For this review, take the finished solid that the model builds, in its own axes (mm). A direction names the side the tool comes from. Coordinates: 2 decimals unless noted, no trailing zeros. Order: outer loops, then holes, each group sorted by start corner. A loop starts at its lowest first (then second) coordinate and runs counter-clockwise, first axis right, second up. Notation, with made-up numbers: M 58,-24.75 L 73,-24.75 A20 ccw 73,3.25 Z; hole C -16,82.25 d4. An arc over 180 degrees is marked long. Use CSV: the item, a comma, the result in double quotes.
Autodesk Inventor part; units mm, degrees
ref_plane "YZ Plane" through (0, 0, 0) normal (1, 0, 0) x (0, 1, 0)
ref_plane "XZ Plane" through (0, 0, 0) normal (0, 1, 0) x (-1, 0, 0)
ref_plane "XY Plane" through (0, 0, 0) normal (0, 0, 1) x (1, 0, 0)
sketch "Sketch1" plane through (0, 0, 0) normal (0, 0, 1) x (1, 0, 0)
  circle A0 centre (10, 20.7) radius 1.6
  line L0 (0, 0) -> (20.0001, 0)
  line L1 (0, 0) -> (0, 7)
  line L2 (20.0001, 0) -> (20.0001, 6.9998)
  line L3 (0, 7) -> (5.4723, 22.0351)
  line L4 (0, 7) -> (16, 7) construction
  line L5 (20.0001, 6.9998) -> (14.5277, 22.0349)
  line L6 (20.0001, 6.9998) -> (36.0001, 6.9998) construction
  arc A1 (14.5277, 22.0349) -> (5.4723, 22.0351) centre (10, 20.3869) ccw
  dimension "d17" = 7
  dimension "d18" = 6.9998
  dimension "d19" = 20.7
  dimension "d23" = 90
  dimension "d24" = 90
  dimension "d25" = 10
  dimension "d26" = 16
  dimension "d27" = 70
  dimension "d28" = 16
  dimension "d29" = 110
  dimension "d30" = 10
sketch "Sketch3" plane through (0, 0, 0) normal (0, 0, 1) x (1, 0, 0)
  point P0 (0, 0)
extrude "Extrusion1" add sketch "Sketch1" along normal blind 4.5
sketch "Sketch4" plane through (0, 0, 4.5) normal (0, 0, 1) x (1, 0, 0)
  line L0 (0, 7) -> (0, 0)
  line L1 (20.0001, 0) -> (20.0001, 6.9998)
  line L2 (0, 0) -> (20.0001, 0)
  line L3 (20.0001, 0) -> (20.0001, 6.9998)
  line L4 (3.884, 22.9404) -> (-0.0481, 7.0119)
  line L5 (20.0001, 6.9998) -> (0, 6.9998)
  line L6 (0, 7) -> (0, 0)
extrude "Extrusion2" add sketch "Sketch4" along normal blind 5.5
sketch "Sketch5" plane through (0, 0, 0) normal (0, -1, 0) x (1, 0, 0)
  circle A0 centre (5, 5) radius 0.5
  circle A1 centre (15, 5) radius 0.5
  point P0 (0, 0)
  dimension "d13" = 1
  dimension "d14" = 1
extrude "Extrusion3" cut sketch "Sketch5" against normal blind 5.5
properties part number "upper_deck_shaft_mount_v2"
Item 1: Add section A-A on z = 1.5. State the section outline as (x, y) points.
Solutions:
outline,"M 0,0 L 20,0 L 20,7 L 14.53,22.03 A4.82 ccw 5.47,22.04 L 0,7 Z; hole C 10,20.7 d3.2"
Item 2: Clearance check with flat-ended pins moving along their axes: pin 1 Ø9 at (x, y) = (5, 14.5) entering from +Z; pin 2 Ø2 at (y, z) = (9, 8.5) entering from -X; pin 3 Ø6 at (x, z) = (14.5, 7) entering from +Y; pin 4 Ø0.8 at (x, z) = (15, 5) entering from -Y. State where each tip first meets the part, or that it passes through.
Solutions:
pin 1,"z = 4.5"
pin 2,"through"
pin 3,"y = 24.28"
pin 4,"y = 5.5"
Item 3: To check wall thickness, follow line 1 along Z through (x, y) = (5, 2.8); line 2 along X through (y, z) = (5, 4.75); line 3 along Y through (x, z) = (10, 1.45). State the ranges of each line that lie inside material, in increasing order. Write a range as [from, to].
Solutions:
line 1,"[0, 4.5], [5.5, 10]"
line 2,"[0, 4.57], [5.43, 14.57], [15.43, 20]"
line 3,"[0, 19.1], [22.3, 25.21]"
Item 4: Add section D-D on z = 5. State the section outline as (x, y) points.
Solutions:
outline,"M 0,0 L 4.5,0 L 4.5,5.5 L 5.5,5.5 L 5.5,0 L 14.5,0 L 14.5,5.5 L 15.5,5.5 L 15.5,0 L 20,0 L 20,7 L 0,7 Z"
Item 5: Add section C-C on y = 20.7. State the section outline as (x, z) points.
Solutions:
outline,"M 4.99,0 L 8.4,0 L 8.4,4.5 L 4.99,4.5 Z; M 11.6,0 L 15.01,0 L 15.01,4.5 L 11.6,4.5 Z"
Item 6: Draft analysis for pull direction Z (two halves, no side actions). For faces 4 (the face through (20, 3, 5)), 5 (the face through (10, 4, 10)), 6 (the face through (15, 5.5, 5)), 7 (the face through (10, 10, 0)), state which applies: released by +Z, released by -Z, zero draft, split by the parting line, or undercut.
Solutions:
face 4,"zero draft"
face 5,"released by +Z"
face 6,"undercut"
face 7,"released by -Z"
Item 7: For faces 1 (the face through (8.73, 21.67, 2.22)), 2 (the face through (10, 14, 4.5)), 3 (the face through (14.935, 2.712, 5.496)), list the 3-axis set-ups (+Z, -Z, +X, -X, +Y, -Y) from which the entire face can be reached by the end or side of a thin tool; tool diameter is ignored.
Solutions:
face 1,"+Z, -Z"
face 2,"+Z, +X, -X, +Y"
face 3,"-Y"
Item 8: Add section B-B on x = 10. State the section outline as (y, z) points, and give its area (3 significant figures).
Solutions:
outline,"M 0,0 L 19.1,0 L 19.1,4.5 L 7,4.5 L 7,10 L 0,10 Z; M 22.3,0 L 25.21,0 L 25.21,4.5 L 22.3,4.5 Z"
area,"138 mm^2"
